Autodesk Inventor part; units mm, degrees
ref_plane "YZ Plane" through (0, 0, 0) normal (1, 0, 0) x (0, 1, 0)
ref_plane "XZ Plane" through (0, 0, 0) normal (0, 1, 0) x (-1, 0, 0)
ref_plane "XY Plane" through (0, 0, 0) normal (0, 0, 1) x (1, 0, 0)
sketch "Sketch1" plane through (0, 0, 0) normal (0, 1, 0) x (-1, 0, 0)
  circle A0 centre (0, 0) radius 84.75
  dimension "d0" = 169.5
extrude "Extrusion1" add sketch "Sketch1" along normal blind 15
sketch "Sketch2" plane through (0, 0, 0) normal (0, -1, 0) x (1, 0, 0)
  circle A0 centre (0, 0) radius 76
  circle A1 centre (0, 76) radius 4
  circle A2 centre (0, -76) radius 4
  circle A3 centre (0, 76) radius 2.25
  circle A4 centre (0, -76) radius 2.25
  dimension "d3" = 152
  dimension "d4" = 8
  dimension "d5" = 8
  dimension "d6" = 4.5
  dimension "d7" = 4.5
extrude "Extrusion2" cut sketch "Sketch2" against normal through all contours A3 A0 | A0 A3 | A4 A0 | A0 A4
extrude "Extrusion3" cut sketch "Sketch2" against normal blind 12 contours A1 A0 A3 | A0 A3 A1 | A2 A0 A4 | A0 A4 A2 | A3 A0 | A0 A3 | A4 A0 | A0 A4
sketch "Sketch3" plane through (0, 0, 0) normal (0, -1, 0) x (1, 0, 0)
  circle A0 centre (0, 0) radius 84.75
  circle A1 centre (0, 0) radius 20
  circle A2 centre (0, -20) radius 4
  circle A3 centre (20, 0) radius 4
  circle A4 centre (0, 20) radius 4
  circle A5 centre (-20, 0) radius 4
  line L0 (55, 55) -> (-55, 55)
  line L1 (-55, 55) -> (-55, -55)
  line L2 (-55, -55) -> (55, -55)
  line L3 (55, -55) -> (55, 55)
  line L4 (55, 55) -> (-55, -55) construction
  line L5 (-55, 55) -> (55, -55) construction
  circle A6 centre (0, 0) radius 55
  circle A7 centre (-38.8909, -38.8909) radius 4
  circle A8 centre (38.8909, -38.8909) radius 4
  circle A9 centre (38.8909, 38.8909) radius 4
  circle A10 centre (-38.8909, 38.8909) radius 4
  dimension "d12" = 40
  dimension "d13" = 8
  dimension "d16" = 360
  dimension "d21" = 110
  dimension "d22" = 110
  dimension "d23" = 110
  dimension "d24" = 8
  dimension "d25" = 8
  dimension "d26" = 8
  dimension "d27" = 8
hole "Hole1" at (38.8909, 0, -38.8909) at (38.8909, 0, 38.8909) at (-38.8909, 0, 38.8909) at (-38.8909, 0, -38.8909) direction (0, 1, 0) diameter 6.647 depth 12 tip angle 118
sketch "Sketch4" plane through (0, 0, 0) normal (0, -1, 0) x (1, 0, 0)
  circle A0 centre (0, 0) radius 45
  circle A1 centre (-45, 0) radius 2.5
  circle A2 centre (-41.5746, -17.2208) radius 2.5
  circle A3 centre (-31.8198, -31.8198) radius 2.5
  circle A4 centre (-17.2208, -41.5746) radius 2.5
  circle A5 centre (0, -45) radius 2.5
  circle A6 centre (17.2208, -41.5746) radius 2.5
  circle A7 centre (31.8198, -31.8198) radius 2.5
  circle A8 centre (41.5746, -17.2208) radius 2.5
  circle A9 centre (45, 0) radius 2.5
  circle A10 centre (41.5746, 17.2208) radius 2.5
  circle A11 centre (31.8198, 31.8198) radius 2.5
  circle A12 centre (17.2208, 41.5746) radius 2.5
  circle A13 centre (0, 45) radius 2.5
  circle A14 centre (-17.2208, 41.5746) radius 2.5
  circle A15 centre (-31.8198, 31.8198) radius 2.5
  circle A16 centre (-41.5746, 17.2208) radius 2.5
  dimension "d35" = 90
  dimension "d36" = 5
  dimension "d39" = 360
hole "Hole2" at (-31.8198, 0, 31.8198) at (31.8198, 0, -31.8198) direction (0, 1, 0) diameter 5 end through all
properties part number "substrate plate"
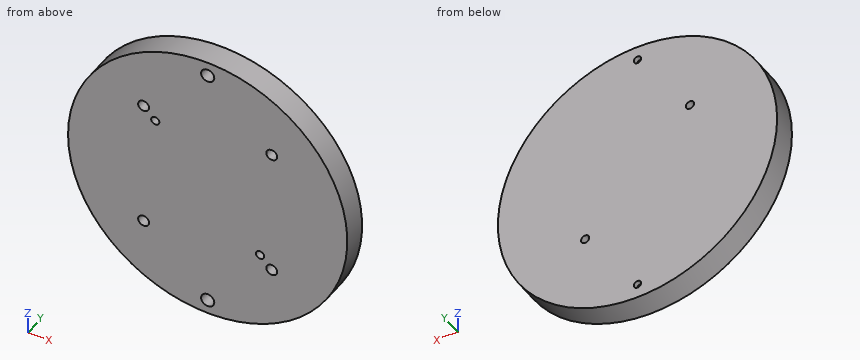
Work out the finished part from the listing and answer in its coordinate system (mm). Give positions to 0.01 mm unless a question says otherwise; leave off trailing zeros. Write each loop counter-clockwise with the first axis right and the second up, starting at its lowest first coordinate (ties: lowest second). Pieces come first, ordered by that corner, then holes. Notation, with made-up numbers: (18.25, 8.25) -> (29.25, 8.25) arc R9 ccw to (29.25, 22.25) -> close; hole circle Ø6 at (-34, 13.5). An arc over 180 degrees is marked (long way). Write item = value, one per line.
Q1. Section D-D on x = -65 is taken. Determine the outline of the cut face in (y, z), and give its area (3 significant figures).
Computed values:
outline = (0, -54.38) -> (15, -54.38) -> (15, 54.38) -> (0, 54.38) -> close
area = 1,630 mm^2
Q2. Section A-A on x = 0 is taken. Determine the outline of the cut face in (y, z).
Computed values:
outline = (0, -84.75) -> (15, -84.75) -> (15, -78.25) -> (12, -78.25) -> (12, -80) -> (0, -80) -> close; (0, -72) -> (12, -72) -> (12, -73.75) -> (15, -73.75) -> (15, 73.75) -> (12, 73.75) -> (12, 72) -> (0, 72) -> close; (0, 80) -> (12, 80) -> (12, 78.25) -> (15, 78.25) -> (15, 84.75) -> (0, 84.75) -> close
Q3. Section B-B on y = 8 is taken. State how many separate pieces and enclosed holes the cut face has, and give its area (3 significant figures).
Computed values:
separate_pieces = 1
enclosed_holes = 8
area = 22,300 mm^2
Q4. Section C-C on z = -76 is taken. Determine the outline of the cut face in (x, y).
Computed values:
outline = (-37.5, 0) -> (-4, 0) -> (-4, 12) -> (-2.25, 12) -> (-2.25, 15) -> (-37.5, 15) -> close; (2.25, 12) -> (4, 12) -> (4, 0) -> (37.5, 0) -> (37.5, 15) -> (2.25, 15) -> close
Q5. Flat-ended cylindrical pins translate along their axes: pin 1 Ø2 at (x, z) = (-62.5, -20.5) entering from -Y; pin 2 Ø6 at (y, z) = (9, 10.5) entering from +X; pin 3 Ø4 at (y, z) = (7, -49) entering from +X; pin 4 Ø4 at (x, z) = (38.89, 38.89) entering from -Y. Find the tip coordinate at first contact, or state that the pin passes through.
Computed values:
pin_1 = 0
pin_2 = 84.42
pin_3 = 70.52
pin_4 = 12.79
Q6. Consider line 1 along Z through (x, y) = (0, 5.75); line 2 along Z through (x, y) = (0, 13.5); line 3 along X through (y, z) = (8, 40). Determine where each line is inside the solid, lowest interval first.
Computed values:
line_1 = -84.75 to -80, -72 to 72, 80 to 84.75
line_2 = -84.75 to -78.25, -73.75 to 73.75, 78.25 to 84.75
line_3 = -74.72 to -42.02, -35.76 to 35.76, 42.02 to 74.72
